CAD build for the part. Positions are in the model's coordinates, mm. A direction names the side the tool comes from. Give positions to 0.01 mm unless a question says otherwise; leave off trailing zeros. Write each loop counter-clockwise with the first axis right and the second up, starting at its lowest first coordinate (ties: lowest second). Pieces come first, ordered by that corner, then holes. Notation, with made-up numbers: (21.25, 15) - (57.25, 15) arc R19 cw to (57.25, 44) - close; hole circle Ø11 at (51.25, 27.5). An arc over 180 degrees is marked (long way). Answer as a JSON object with one key per item and string values.
from build123d import *

# Parameters (mm, degrees)
SKETCH3_W           = 39
SKETCH3_H           = 70.3
SKETCH3_R           = 1.5
SKETCH3_W_2         = 12.7
SKETCH3_H_2         = 32.4
BOSS_EXTRUDE1_DEPTH = 2
FILLET1_R           = 3


with BuildPart() as part:
    # Sketch3 → Boss-Extrude1 (new body)
    with BuildSketch(Plane(origin=(0, 0, 0), x_dir=(1, 0, 0), z_dir=(0, 1, 0))):
        with Locations((0, 4.534618943)):
            Rectangle(SKETCH3_W, SKETCH3_H)
        with Locations(Location((-7.25, 35.459618943, 0), (0, 0, 270))):
            Circle(SKETCH3_R, mode=Mode.SUBTRACT)
        with Locations(Location((7.25, 35.459618943, 0), (0, 0, 270))):
            Circle(SKETCH3_R, mode=Mode.SUBTRACT)
        with Locations(Location((7.25, -26.390381057, 0), (0, 0, 270))):
            Circle(SKETCH3_R, mode=Mode.SUBTRACT)
        with Locations(Location((-7.25, -26.390381057, 0), (0, 0, 270))):
            Circle(SKETCH3_R, mode=Mode.SUBTRACT)
        with Locations(Location((9.175, 26.675, 0), (0, 0, 270))):
            Circle(SKETCH3_R, mode=Mode.SUBTRACT)
        with Locations(Location((9.175, -9.025, 0), (0, 0, 270))):
            Circle(SKETCH3_R, mode=Mode.SUBTRACT)
        with Locations(Location((-9.175, 26.675, 0), (0, 0, 270))):
            Circle(SKETCH3_R, mode=Mode.SUBTRACT)
        with Locations(Location((-9.175, -9.025, 0), (0, 0, 270))):
            Circle(SKETCH3_R, mode=Mode.SUBTRACT)
        with Locations((0, 5.2)):
            Rectangle(SKETCH3_W_2, SKETCH3_H_2, mode=Mode.SUBTRACT)
    extrude(amount=-BOSS_EXTRUDE1_DEPTH)

    # Fillet1
    fillet1_edges = [part.edges().sort_by_distance(p)[0] for p in [
        (-19.5, -1, -39.684618943),
        (19.5, -1, -39.684618943),
        (19.5, -1, 30.615381057),
        (-19.5, -1, 30.615381057),
    ]]
    fillet(fillet1_edges, radius=FILLET1_R)


solid = part.part
(1) Saw through at B-B, the plane y = -0.6. State how many separate pieces and enclosed holes the cut face has, and give its area (3 significant figures).
Answer key:
{"separate pieces": "1", "enclosed holes": "9", "area": "2,270 mm²"}
(2) Saw through at A-A, the plane z = -15.5. Give the cut face in (x, y).
Answer key:
{"outline": "(-19.5, -2) - (-6.35, -2) - (-6.35, 0) - (-19.5, 0) - close; (6.35, -2) - (19.5, -2) - (19.5, 0) - (6.35, 0) - close"}
(3) 3-axis set-ups, long thin cutter, end or side, ignore diameter. For faces 1 (the face through (0, -1, -21.4)), 2 (the face through (18.598, -1.014, -38.829)): which of +Z, -Z, +X, -X, +Y, -Y reach the whole face in a straight line?
Answer key:
{"face 1": "+Y, -Y", "face 2": "-Z, +X, +Y, -Y"}
(4) Probe L1, parallel to X at y = -0.1, z = 9; L2, parallel to X at y = -1.6, z = -12.5; L3, parallel to Z at x = -1.5, y = -1.5. List the from-to ranges inside material, lowest first. Write a range as [from, to].
Answer key:
{"L1": "x = [-19.5, -10.67], [-7.68, -6.35], [6.35, 7.68], [10.67, 19.5]", "L2": "x = [-19.5, -6.35], [6.35, 19.5]", "L3": "z = [-39.68, -21.4], [11, 30.62]"}
(5) Pull direction X, two halves, no side cores. Call faces 3 (the face through (0, -1, 30.615)), 4 (the face through (0, -1, 11)), 5 (the face through (-18.645, -1.014, -38.782)): pulls with the +X half, pulls with the -X half, needs draft (parallel to the pull), parting line crosses it, or undercut.
Answer key:
{"face 3": "needs draft", "face 4": "undercut", "face 5": "pulls with the -X half"}
